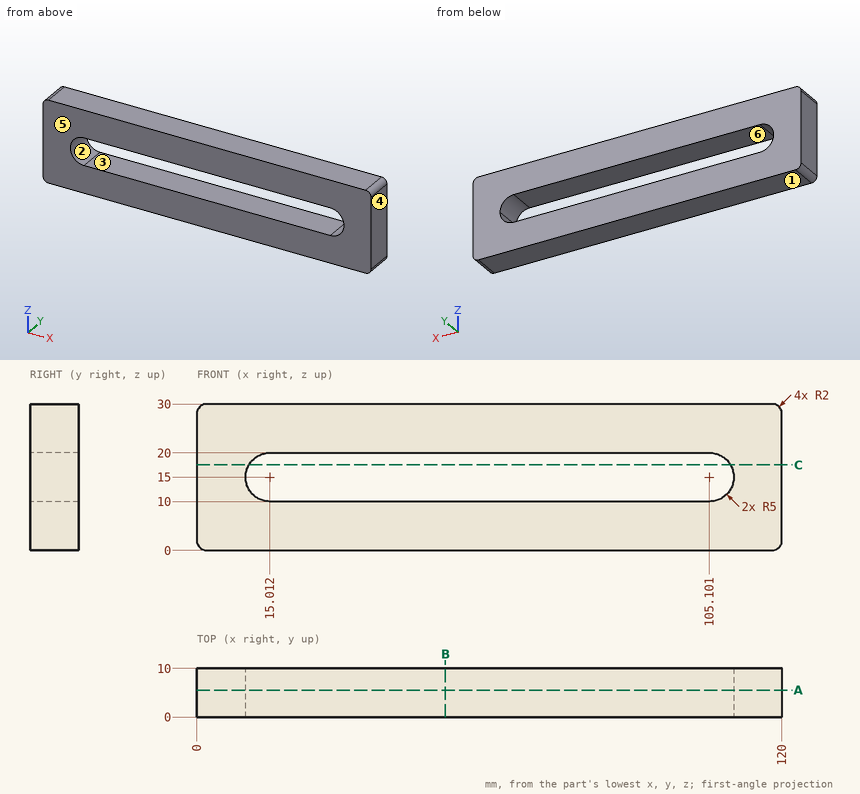
Part print with two shaded views. Sizes in mm from the minimum x, y, z corner. A direction names the side the tool comes from. Round coordinates to 2 decimals unless told otherwise and drop trailing zeros. Order: outer loops, then holes, each group sorted by start corner. A loop starts at its lowest first (then second) coordinate and runs counter-clockwise, first axis right, second up. Notation, with made-up numbers: M 78,28.5 L 133,28.5 A38 cw 133,67.5 Z; hole C -33.75,-8.5 d2. An arc over 180 degrees is marked long. Put each result on its own line as item: value. Start each with the question number.
1. Tool access for the marked faces 1 and 2: list every direction of +Z, -Z, +X, -X, +Y, -Y with a clear straight run to the whole face (end or side of a thin tool).
2. Slice it at A-A on y = 5.5. List the corners of the cut face in (x, z), then the cut area to 3 significant figures.
3. Drill centre lines: probe 1 along Z at (x, y) = (79.5, 9.5); probe 2 along X at (y, z) = (4.25, 11); probe 3 along Z at (x, y) = (107.5, 7.75). Where is each one in solid material? Low to high. Write a range as [from, to].
4. Slice it at B-B on x = 51. List the corners of the cut face in (y, z).
5. Drop a flat-ended pin along its axis: pin 1 (8 mm diameter, centred on x = 83.5, z = 26.5, fed in from -Y). Give the stop position or say it passes through.
6. Two-plate mould, pull along X, no slides. Class the marked faces 3, 4, 5 and 6: +X half, -X half, draft (parallel to the pull), parting line (faces both ways), or undercut.
7. Slice it at C-C on z = 17.5. List the corners of the cut face in (x, y).
Findings:
1. face 1: -Z, +X, -X, +Y, -Y
1. face 2: +Y, -Y
2. outline: M 0,2 A2 ccw 2,0 L 118,0 A2 ccw 120,2 L 120,28 A2 ccw 118,30 L 2,30 A2 ccw 0,28 Z; hole M 15.01,10 L 105.1,10 A5 ccw 105.1,20 L 15.01,20 A5 ccw Z
2. area: 2,620 mm2
3. probe 1: [0, 10], [20, 30]
3. probe 2: [0, 12.01], [108.1, 120]
3. probe 3: [0, 10.61], [19.39, 30]
4. outline: M 0,0 L 10,0 L 10,10 L 0,10 Z; M 0,20 L 10,20 L 10,30 L 0,30 Z
5. pin 1: y = 0
6. face 3: undercut
6. face 4: +X half
6. face 5: draft
6. face 6: undercut
7. outline: M 0,0 L 10.68,0 L 10.68,10 L 0,10 Z; M 109.43,0 L 120,0 L 120,10 L 109.43,10 Z
